CAD build for the part. Positions are in the model's coordinates, mm. A direction names the side the tool comes from. Give positions to 0.01 mm unless a question says otherwise; leave off trailing zeros. Loops run counter-clockwise (first coordinate to the right, second up) from the corner with the lowest first, then second, coordinate; pieces in that order, holes last. Notation, with made-up numbers: M -4,77 L 9,77 A10 ccw 9,93 Z; hole C 0.5,-17.5 d10. An arc over 180 degrees is marked long. Answer as CSV lines item,"result".
from build123d import *

# Parameters (mm, degrees)
SKETCH1_W           = 20
SKETCH1_H           = 20
SKETCH1_W_2         = 16
SKETCH1_H_2         = 16
BOSS_EXTRUDE1_DEPTH = 480
SKETCH2_R           = 2.5
CUT_EXTRUDE1_DEPTH  = 481.520551069
SKETCH3_R           = 2.5
CUT_EXTRUDE2_DEPTH  = 481.520551069
SKETCH4_R           = 2.5
CUT_EXTRUDE3_DEPTH  = 20


with BuildPart() as part:
    # Sketch1 → Boss-Extrude1 (new body)
    with BuildSketch(Plane(origin=(0, 0, 0), x_dir=(0, 0, -1), z_dir=(1, 0, 0))):
        Rectangle(SKETCH1_W, SKETCH1_H)
        Rectangle(SKETCH1_W_2, SKETCH1_H_2, mode=Mode.SUBTRACT)
    extrude(amount=BOSS_EXTRUDE1_DEPTH)

    # Sketch2 → Cut-Extrude1 (cut, through all)
    with BuildSketch(Plane(origin=(0, 10, 0), x_dir=(1, 0, 0), z_dir=(0, 1, 0))):
        with Locations(Location((10, 0, 0), (0, 0, 270))):
            Circle(SKETCH2_R)
        with Locations(Location((470, 0, 0), (0, 0, 270))):
            Circle(SKETCH2_R)
        with Locations(Location((25, 0, 0), (0, 0, 270))):
            Circle(SKETCH2_R)
        with Locations(Location((455, 0, 0), (0, 0, 270))):
            Circle(SKETCH2_R)
    extrude(amount=-CUT_EXTRUDE1_DEPTH, mode=Mode.SUBTRACT)

    # Sketch3 → Cut-Extrude2 (cut, through all)
    with BuildSketch(Plane(origin=(0, 10, 0), x_dir=(1, 0, 0), z_dir=(0, 1, 0))):
        with Locations(Location((175, 0, 0), (0, 0, 270))):
            Circle(SKETCH3_R)
        with Locations(Location((305, 0, 0), (0, 0, 270))):
            Circle(SKETCH3_R)
        with Locations(Location((205, 0, 0), (0, 0, 270))):
            Circle(SKETCH3_R)
        with Locations(Location((275, 0, 0), (0, 0, 270))):
            Circle(SKETCH3_R)
    extrude(amount=-CUT_EXTRUDE2_DEPTH, mode=Mode.SUBTRACT)

    # Sketch4 → Cut-Extrude3 (cut)
    with BuildSketch(Plane.XY.offset(10)):
        with Locations((60, 0)):
            Circle(SKETCH4_R)
        with Locations((90, 0)):
            Circle(SKETCH4_R)
        with Locations((315, 0)):
            Circle(SKETCH4_R)
        with Locations((345, 0)):
            Circle(SKETCH4_R)
        with Locations((135, 0)):
            Circle(SKETCH4_R)
        with Locations((155, 0)):
            Circle(SKETCH4_R)
        with Locations((230, 0)):
            Circle(SKETCH4_R)
        with Locations((250, 0)):
            Circle(SKETCH4_R)
    extrude(amount=-CUT_EXTRUDE3_DEPTH, mode=Mode.SUBTRACT)


solid = part.part
1) Which spindle directions (+Z, -Z, +X, -X, +Y, -Y) get a long thin tool onto all of the face, cutting with end or side? Do faces 4 (the face through (237, 8, 0)), 5 (the face through (237, 10, 0)). Say none if no direction does.
Answer below:
face 4,"+X, -X"
face 5,"+Z, -Z, +X, -X, +Y"
2) Drill centre lines: line 1 (Z direction, x = 305, y = 9.1); line 2 (Z direction, x = 345, y = 3.5). Where is each one in solid material? Low to high. Write a range as from..to.
Answer below:
line 1,"z = -10..-2.5, 2.5..10"
line 2,"z = -10..-8, 8..10"
3) Band-saw the part on A-A on x = 186.5. Give the cut face in (y, z), and give its area (3 significant figures).
Answer below:
outline,"M -10,-10 L 10,-10 L 10,10 L -10,10 Z; hole M -8,-8 L 8,-8 L 8,8 L -8,8 Z"
area,"144 mm^2"
4) Mould opens along Z. For faces 1 (the face through (237, -10, 0)), 2 (the face through (237, 0, -10)), 3 (the face through (237, 0, -8)) say: +Z half, -Z half, draft (parallel to the pull), parting line (faces both ways), or undercut.
Answer below:
face 1,"draft"
face 2,"-Z half"
face 3,"undercut"
